```python
from build123d import *

# Parameters (mm, degrees)
F0_W     = 3.8
F0_H     = 3.840202
F0_H_2   = 3.959798
F1_DEPTH = 10
F2_W     = 3.8
F2_H     = 3.840202
F3_DEPTH = 6
F4_R     = 5.5
F5_DEPTH = 5
F6_R     = 1
F7_DEPTH = 25
F8_R     = 4.2
F9_DEPTH = 14
F10_R    = 7


with BuildPart() as f1:
    # F0 (on Top) → F1 (new body)
    with BuildSketch(Plane.XY):
        Polygon((0, 15), (0, 0), (15, 0), (15, 15), (9.4, 15), (5.6, 15), align=None)
        with Locations((7.5, 16.920101)):
            Rectangle(F0_W, F0_H)
        with Locations((7.5, 20.820101)):
            Rectangle(F0_W, F0_H_2)
        Polygon((9.4, 22.8), (9.4, 18.840202), (14.066905, 23.507107), (12.087006, 25.487006), align=None)
        Polygon((0.933095, 23.507107), (5.6, 18.840202), (5.6, 22.8), (2.912994, 25.487006), align=None)
    extrude(amount=F1_DEPTH)

    # F2 (on face) → F3 (join)
    with BuildSketch(Plane.XY.offset(10)):
        with Locations((7.5, 16.920101)):
            Rectangle(F2_W, F2_H)
    extrude(amount=F3_DEPTH)

    # F4 (on face) → F5 (join)
    with BuildSketch(Plane(origin=(0, 0, 0), x_dir=(1, 0, 0), z_dir=(0, 0, -1))):
        with Locations((7.5, -7.5)):
            Circle(F4_R)
    extrude(amount=F5_DEPTH)

    # F6 (on face) → F7 (cut)
    with BuildSketch(Plane(origin=(0, 0, -5), x_dir=(1, 0, 0), z_dir=(0, 0, -1))):
        with Locations((7.5, -7.5)):
            Circle(F6_R)
    extrude(amount=-F7_DEPTH, mode=Mode.SUBTRACT)

    # F8 (on face) → F9 (cut)
    with BuildSketch(Plane.XY.offset(10)):
        with Locations((7.5, 7.5)):
            Circle(F8_R)
    extrude(amount=-F9_DEPTH, mode=Mode.SUBTRACT)

    # F10
    f10_edges = [f1.edges().sort_by_distance(p)[0] for p in [
        (15, 0, 5),
        (0, 0, 5),
    ]]
    fillet(f10_edges, radius=F10_R)


solid = f1.part
```
The model under review builds one solid part; all positions refer to its coordinate system, in mm. A direction names the side the tool comes from. Round coordinates to 2 decimals unless told otherwise and drop trailing zeros. Order: outer loops, then holes, each group sorted by start corner. A loop starts at its lowest first (then second) coordinate and runs counter-clockwise, first axis right, second up. Notation, with made-up numbers: (65.25, 2.25) - (122.25, 2.25) arc R20 ccw to (122.25, 30.25) - close; hole circle Ø5 at (-32.5, -10.5). An arc over 180 degrees is marked (long way). Answer in a Markdown table with one row per item.
(1) Take a section at B-B on z = 5.75. Write out the cut boundary in (x, y).
Result set:
| item | result |
|---|---|
| outline | (0, 7) arc R7 ccw to (7, 0) - (8, 0) arc R7 ccw to (15, 7) - (15, 15) - (9.4, 15) - (9.4, 18.84) - (14.07, 23.51) - (12.09, 25.49) - (9.4, 22.8) - (5.6, 22.8) - (2.91, 25.49) - (0.93, 23.51) - (5.6, 18.84) - (5.6, 15) - (0, 15) - close; hole circle Ø8.4 at (7.5, 7.5) |
(2) For line 1 (Y direction, x = 7.5, z = -4.5); line 2 (Y direction, x = 7.75, z = 0.25); line 3 (Y direction, x = 4.5, z = 9), list the stretches that pass through material, from the lowest coordinate up. Write a range as from..to.
Result set:
| item | result |
|---|---|
| line 1 | y = 2..6.5, 8.5..13 |
| line 2 | y = 0..3.31, 11.69..22.8 |
| line 3 | y = 0.46..4.56, 10.44..15, 19.94..23.9 |
(3) Take a section at A-A on x = 7.5. Write out the cut boundary in (y, z).
Result set:
| item | result |
|---|---|
| outline | (0, 0) - (2, 0) - (2, -5) - (6.5, -5) - (6.5, -4) - (3.3, -4) - (3.3, 10) - (0, 10) - close; (8.5, -5) - (13, -5) - (13, 0) - (22.8, 0) - (22.8, 10) - (18.84, 10) - (18.84, 16) - (15, 16) - (15, 10) - (11.7, 10) - (11.7, -4) - (8.5, -4) - close |
(4) Clearance check with flat-ended pins moving along their axes: P1, Ø4, axis at y = 17, z = 10.5, coming from the +X side; P2, Ø3, axis at y = 16.5, z = 11, coming from the -X side; P3, Ø4, axis at x = 10, z = 1.5, coming from the +Y side. State where each tip first meets the part, or that it passes through.
Result set:
| item | result |
|---|---|
| P1 | stops at x = 9.5 |
| P2 | stops at x = 5.6 |
| P3 | stops at y = 25.4 |
(5) Take a section at D-D on x = 12.5. Write out the cut boundary in (y, z), plus the area to 3 significant figures.
Result set:
| item | result |
|---|---|
| outline | (1.64, 0) - (5.21, 0) - (5.21, -5) - (9.79, -5) - (9.79, 0) - (15, 0) - (15, 10) - (1.64, 10) - close; (21.94, 0) - (25.07, 0) - (25.07, 10) - (21.94, 10) - close |
| area | 188 mm2 |
(6) Take a section at C-C on y = 7.5. Write out the cut boundary in (x, z).
Result set:
| item | result |
|---|---|
| outline | (0, 0) - (2, 0) - (2, -5) - (6.5, -5) - (6.5, -4) - (3.3, -4) - (3.3, 10) - (0, 10) - close; (8.5, -5) - (13, -5) - (13, 0) - (15, 0) - (15, 10) - (11.7, 10) - (11.7, -4) - (8.5, -4) - close |
(7) Mouldability with a two-part tool opening along X and no side actions: class faces 5 (the face through (8.4, 6.6, -4)), 6 (the face through (3.23, 21.21, 4.93)), 7 (the face through (10.8, 24.2, 4.9)), 8 (the face through (9, 13, 0)) as released by +X, released by -X, zero draft, split by the parting line, or undercut.
Result set:
| item | result |
|---|---|
| face 5 | undercut |
| face 6 | released by -X |
| face 7 | undercut |
| face 8 | zero draft |
(8) Machinability: for faces 1 (the face through (9.438, 3.774, 3.098)), 2 (the face through (7, 22, 10)), 3 (the face through (3, 15, 5)), 4 (the face through (6.31, 12.87, -2.46)), which of the approach directions +Z, -Z, +X, -X, +Y, -Y give a long, thin tool a straight path to every point of the face, cutting with its end or side? Answer none if there is none.
Result set:
| item | result |
|---|---|
| face 1 | +Z |
| face 2 | +Z, +X, -X, +Y |
| face 3 | +Z, -Z, -X |
| face 4 | -Z |
